Job drawing, mm, ordinate dimensions from the low corner. One solid piece. A direction names the side the tool comes from. Give positions to 0.01 mm unless a question says otherwise; leave off trailing zeros. Write each loop counter-clockwise with the first axis right and the second up, starting at its lowest first coordinate (ties: lowest second). Pieces come first, ordered by that corner, then holes. Notation, with made-up numbers: M 16.5,70 L 61.5,70 A30 ccw 61.5,106 Z; hole C -40,18.5 d3. An arc over 180 degrees is marked long. Answer as CSV lines item,"result". Start each with the question number.
Item 1: Band-saw the part on D-D, the plane x = 55. List the corners of the cut face in (y, z), then the cut area to 3 significant figures.
Item 2: Band-saw the part on A-A, the plane y = 9. List the corners of the cut face in (x, z).
Item 3: Wall check: L1, parallel to Y at x = 52, z = 9.5; L2, parallel to Y at x = 56.5, z = 42; L3, parallel to Z at x = 44, y = 19. Give the ranges that are in metal, low to high. Write a range as from..to.
Item 4: Band-saw the part on B-B, the plane z = 10. List the corners of the cut face in (x, y), then the cut area to 3 significant figures.
Item 5: 3-axis set-ups, long thin cutter, end or side, ignore diameter. For the marked faces 5 and 6: which of +Z, -Z, +X, -X, +Y, -Y reach the whole face in a straight line?
Item 6: Two-plate mould, pull along X, no slides. Class the marked faces 1, 2, 3 and 4: +X half, -X half, draft (parallel to the pull), parting line (faces both ways), or undercut.
Item 7: Band-saw the part on C-C, the plane y = 31. List the corners of the cut face in (x, z), then the cut area to 3 significant figures.
Item 8: Pin check, flat tips, straight feed: pin 1 (1.5 mm diameter, centred on x = 37, y = 29.5, fed in from +Z); pin 2 (4 mm diameter, centred on x = 44.5, z = 9.5, fed in from -Y); pin 3 (8 mm diameter, centred on x = 40.5, z = 19.5, fed in from -Y). Stop position of each tip, or through.
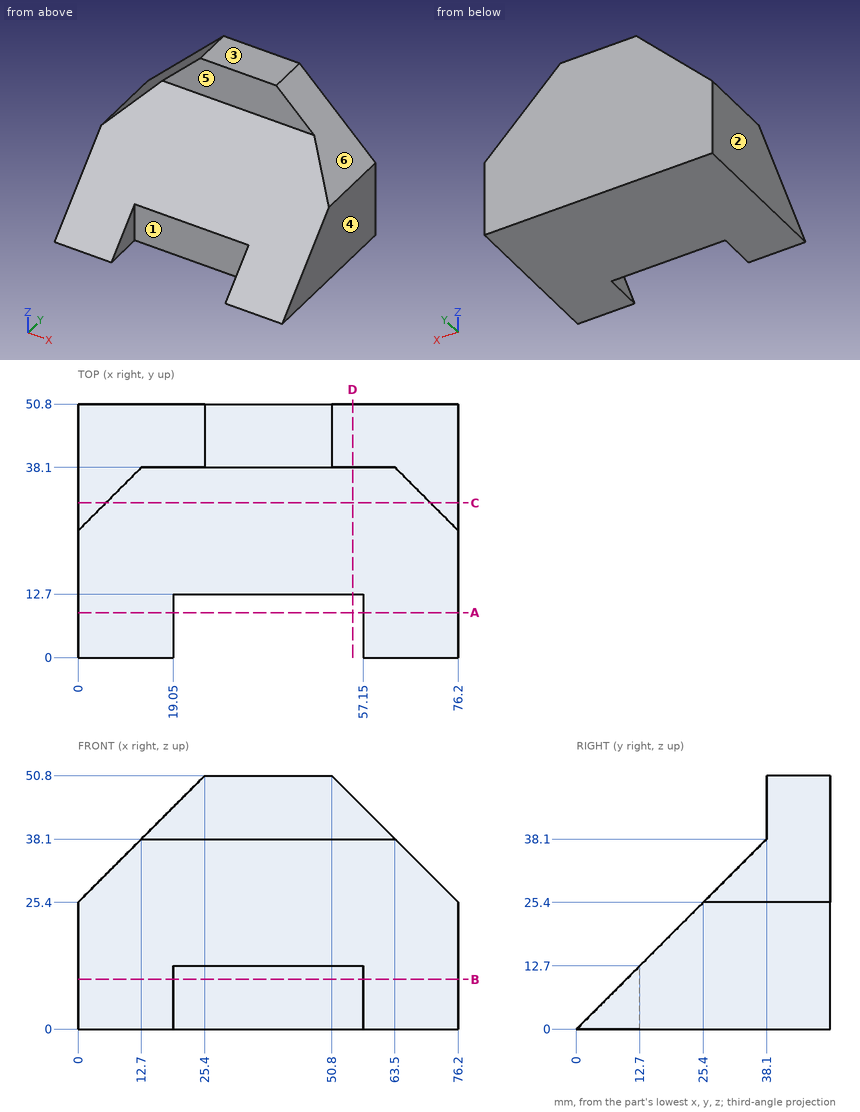
Output:
1,outline,"M 12.7,0 L 50.8,0 L 50.8,46.6 L 38.1,46.6 L 38.1,38.1 L 12.7,12.7 Z"
1,area,"1,240 mm²"
2,outline,"M 0,0 L 19.05,0 L 19.05,9 L 0,9 Z; M 57.15,0 L 76.2,0 L 76.2,9 L 57.15,9 Z"
3,L1,"12.7..50.8"
3,L2,"38.1..50.8"
3,L3,"0..19"
4,outline,"M 0,10 L 19.05,10 L 19.05,12.7 L 57.15,12.7 L 57.15,10 L 76.2,10 L 76.2,50.8 L 0,50.8 Z"
4,area,"3,010 mm²"
5,face 5,"+Z, +X, -X, -Y"
5,face 6,"+Z, +X, +Y, -Y"
6,face 1,"undercut"
6,face 2,"-X half"
6,face 3,"draft"
6,face 4,"+X half"
7,outline,"M 0,0 L 76.2,0 L 76.2,25.4 L 70.6,31 L 5.6,31 L 0,25.4 Z"
7,area,"2,330 mm²"
8,pin 1,"z = 30.25"
8,pin 2,"y = 12.7"
8,pin 3,"y = 15.5"
